Geometry: final body of the model. Coordinates: model frame, mm. A direction names the side the tool comes from. Round coordinates to 2 decimals unless told otherwise and drop trailing zeros. Loops run counter-clockwise (first coordinate to the right, second up) from the corner with the lowest first, then second, coordinate; pieces in that order, holes last. Notation, with made-up numbers: (-8.5, 19) - (18.5, 19) arc R23 ccw to (18.5, 32) - close; hole circle Ø10 at (-9, 26). An arc over 180 degrees is marked (long way). Answer in a Markdown table with one row per item. Add a question column.
Autodesk Inventor part; units mm, degrees
ref_plane "YZ Plane" through (0, 0, 0) normal (1, 0, 0) x (0, 1, 0)
ref_plane "XZ Plane" through (0, 0, 0) normal (0, 1, 0) x (-1, 0, 0)
ref_plane "XY Plane" through (0, 0, 0) normal (0, 0, 1) x (1, 0, 0)
sketch "스케치1" plane through (0, 0, 0) normal (0, 1, 0) x (-1, 0, 0)
  line L0 (0, 0) -> (0, -15.6)
  line L1 (0, -15.6) -> (18, -15.6)
  line L2 (0, 0) -> (15, 0)
  line L3 (15, 0) -> (15, -1.3)
  line L4 (15, -1.3) -> (5, -1.3)
  line L5 (5, -1.3) -> (5, -5.3)
  line L6 (5, -5.3) -> (4, -5.3)
  line L7 (4, -5.3) -> (4, -9.3)
  line L8 (4, -9.3) -> (5, -9.3)
  line L9 (5, -9.3) -> (5, -13.3)
  line L10 (5, -13.3) -> (18, -13.3)
  line L11 (18, -13.3) -> (18, -15.6)
  line L12 (3, 0) -> (19.1, 0) construction
  line L13 (19.1, 0) -> (19.1, -14.6) construction
  line L14 (19.1, -14.6) -> (3, -14.6) construction
  line L15 (3, -14.6) -> (3, 0) construction
  line L16 (19.1, -7.3) -> (3, -7.3) construction
  dimension "d0" = 15.6
  dimension "d1" = 18
  dimension "d2" = 15
  dimension "d3" = 1.3
  dimension "d4" = 10
  dimension "d5" = 4
  dimension "d6" = 1
  dimension "d7" = 4
  dimension "d8" = 1
  dimension "d9" = 4
  dimension "d10" = 13
  dimension "d18" = 16.1
  dimension "d19" = 14.6
  dimension "d20" = 3
  dimension "d21" = 1
extrude "돌출1" add sketch "스케치1" along normal blind 4
sketch "스케치2" plane through (-15, 0, 0) normal (0, 0, 1) x (1, 0, 0)
  line L0 (-3, 1.5) -> (12, 1.5)
  line L1 (12, 1.5) -> (12, 2.5)
  line L2 (12, 2.5) -> (-3, 2.5)
  line L3 (-3, 2.5) -> (-3, 1.5)
  line L4 (15, 0) -> (15, 4)
  line L5 (0, 0) -> (0, 4)
  line L6 (0, 0) -> (15, 0)
  line L7 (-3, 0) -> (-3, 4)
  dimension "d13" = 1
  dimension "d14" = 3
  dimension "d15" = 1.5
extrude "돌출2" cut sketch "스케치2" against normal blind 14.6
sketch "스케치3" plane through (0, 4, 0) normal (0, 1, 0) x (1, 0, 0)
  line L0 (0, 0) -> (0, 15.6)
  line L1 (0, 15.6) -> (-18, 15.6)
  line L2 (0, 0) -> (-4, 0)
  line L3 (-4, 0) -> (-4, 13)
  line L4 (-4, 13) -> (0, 13)
  line L5 (0, 13) -> (0, 0)
  line L6 (-15, 0) -> (0, 0)
  point P0 (-3, 0)
  dimension "d22" = 4
  dimension "d23" = 13
extrude "돌출3" add sketch "스케치3" along normal blind 2
sketch "스케치4" plane through (0, 6, 0) normal (0, 1, 0) x (1, 0, 0)
  line L0 (0, 0) -> (0, 15.6)
  line L1 (-4, 13) -> (0, 13)
  line L2 (0, 13) -> (0, 11)
  line L3 (0, 11) -> (-4, 11)
  line L4 (-4, 11) -> (-4, 13)
  line L5 (0, 0) -> (0, 13)
  line L6 (0, 13) -> (-4, 13)
  line L7 (-4, 13) -> (-4, 0)
  line L8 (-4, 0) -> (0, 0)
  dimension "d26" = 2
extrude "돌출4" add sketch "스케치4" along normal blind 4 contours L3 L4 L1 L0
sketch "스케치5" plane through (0, 4, 0) normal (0, 1, 0) x (1, 0, 0)
  line L0 (-4, 0) -> (-4, 5.3)
  line L1 (-4, 5.3) -> (-5, 5.3)
  line L2 (-5, 5.3) -> (-5, 1.3)
  line L3 (-5, 1.3) -> (-15, 1.3)
  line L4 (-15, 1.3) -> (-15, 0)
  line L5 (-15, 0) -> (-4, 0)
  line L6 (-4, 9.3) -> (-4, 13)
  line L7 (-4, 13) -> (0, 13)
  line L8 (0, 13) -> (0, 15.6)
  line L9 (0, 15.6) -> (-18, 15.6)
  line L10 (-18, 15.6) -> (-18, 13.3)
  line L11 (-18, 13.3) -> (-5, 13.3)
  line L12 (-5, 13.3) -> (-5, 9.3)
  line L13 (-5, 9.3) -> (-4, 9.3)
  line L14 (-4, 0) -> (-5, 0)
  line L15 (-5, 0) -> (-5, 13)
  line L16 (-5, 13) -> (-4, 13)
  line L17 (-4, 13) -> (-4, 0)
  point P0 (0, 0)
  dimension "d31" = 13
extrude "돌출5" add sketch "스케치5" along normal blind 2 contours L5 L15 L2 L1 L0 | L1 L15 L13 L17 | L5 L4 L3 L15 | L13 L12 L16 L6
properties part number "PCB_Holder"
1) Contact query for flat-ended pins moving along their axis: pin 1 Ø2 at (x, y) = (-12.5, 7.5) entering from +Z; pin 2 Ø2 at (y, z) = (8, -12.5) entering from -X; pin 3 Ø1.5 at (x, z) = (-6, -13.5) entering from +Y; pin 4 Ø1.4 at (y, z) = (1, -0.5) entering from -X. Output: stop coordinate, or through.
2) Section B-B, the plane x = -4.5. Return the cut outline in (y, z).
3) Material intervals for line 1 along Z through (x, y) = (-12.5, 3); line 2 along Y through (x, z) = (-4.75, -3); line 3 along Y through (x, z) = (-8, -14.5), sorted ascending. Write a range as from..to.
4) Reachability of faces 1 (the flat face through (-15, 4, -1)), 2 (the flat face through (-2, 7, -13)), 3 (the flat face through (-4.5, 3.2, -9.3)), 4 (the flat face through (-5, 4.2, -7.2)), 5 (the flat face through (-4, 1.5, -10)) from +Z, -Z, +X, -X, +Y, -Y: full face, straight path, thin tool, end or side. Return the list, or none.
5) Section C-C, the plane z = -6. Return the cut outline in (x, y), and give its area (3 significant figures).
6) Section A-A, the plane x = -12. Return the cut outline in (y, z), and give its area (3 significant figures).
7) Section D-D, the plane y = 5.5. Return the cut outline in (x, z), and give its area (3 significant figures).
8) Pull-direction query (Y, two-part tool) for faces 6 (the flat face through (-11, 2, -14.6)), 7 (the flat face through (-18, 2, -15)), 8 (the flat face through (-3, 2, -7)), 9 (the flat face through (-4.5, 4, -7.3)); classes: pulls with the +Y half, pulls with the -Y half, needs draft (parallel to the pull), parting line crosses it, or undercut.
Evaluation:
| question | item | result |
|---|---|---|
| 1 | pin 1 | passes through |
| 1 | pin 2 | stops at x = -4 |
| 1 | pin 3 | stops at y = 4 |
| 1 | pin 4 | stops at x = -15 |
| 2 | outline | (0, -15.6) - (4, -15.6) - (4, -13) - (6, -13) - (6, 0) - (2.5, 0) - (2.5, -5.3) - (4, -5.3) - (4, -9.3) - (2.5, -9.3) - (2.5, -14.6) - (1.5, -14.6) - (1.5, -9.3) - (0, -9.3) - close; (0, -5.3) - (1.5, -5.3) - (1.5, 0) - (0, 0) - close |
| 3 | line 1 | z = -15.6..-13.3, -1.3..0 |
| 3 | line 2 | y = 0..1.5, 2.5..6 |
| 3 | line 3 | y = 0..1.5, 2.5..4 |
| 4 | face 1 | +Z, -X, +Y, -Y |
| 4 | face 2 | -Z, +X, -X, +Y |
| 4 | face 3 | -X, -Y |
| 4 | face 4 | -X, +Y, -Y |
| 4 | face 5 | +Z, -X |
| 5 | outline | (-5, 4) - (-4, 4) - (-4, 2.5) - (-3, 2.5) - (-3, 1.5) - (-4, 1.5) - (-4, 0) - (0, 0) - (0, 6) - (-5, 6) - close |
| 5 | area | 25.0 mm² |
| 6 | outline | (0, -15.6) - (4, -15.6) - (4, -13.3) - (2.5, -13.3) - (2.5, -14.6) - (1.5, -14.6) - (1.5, -13.3) - (0, -13.3) - close; (0, -1.3) - (1.5, -1.3) - (1.5, 0) - (0, 0) - close; (2.5, -1.3) - (6, -1.3) - (6, 0) - (2.5, 0) - close |
| 6 | area | 14.4 mm² |
| 7 | outline | (-15, -1.3) - (-5, -1.3) - (-5, -13) - (0, -13) - (0, 0) - (-15, 0) - close |
| 7 | area | 78.0 mm² |
| 8 | face 6 | undercut |
| 8 | face 7 | needs draft |
| 8 | face 8 | undercut |
| 8 | face 9 | pulls with the -Y half |
